from build123d import *

# Parameters (mm, degrees)
ESBO_O1_R                = 7.65
RESSALTO_EXTRUS_O1_DEPTH = 26
ESBO_O4_R                = 1.75
CORTE_EXTRUS_O1_DEPTH    = 20
ESBO_O5_W                = 3
ESBO_O5_H                = 5.6
CORTE_EXTRUS_O2_DEPTH    = 25
RESSALTO_EXTRUS_O2_DEPTH = 13
ESBO_O7_R                = 9
CORTE_EXTRUS_O3_DEPTH    = 10


with BuildPart() as part:
    # Esboço1 → Ressalto-extrusão1 (new body)
    with BuildSketch(Plane.XY):
        with BuildLine():
            Line((-7, 20.253205655), (-7, 18.253205655))
            Line((-7, 18.253205655), (-47, 18.253205655))
            Line((-47, 18.253205655), (-47, 8.253205655))
            Line((-47, 8.253205655), (-7, 8.253205655))
            Line((-7, 8.253205655), (-7, -20.253205655))
            ThreePointArc((-7, -20.253205655), (3.676851089, -41.422817781), (0, -18))
            Line((0, -18), (0, 18))
            ThreePointArc((0, 18), (3.676851089, 41.422817781), (-7, 20.253205655))
        make_face()
        with Locations(Location((0, 30, 0), (0, 0, 180))):
            Circle(ESBO_O1_R, mode=Mode.SUBTRACT)
        with Locations(Location((0, -30, 0), (0, 0, 180))):
            Circle(ESBO_O1_R, mode=Mode.SUBTRACT)
    extrude(amount=RESSALTO_EXTRUS_O1_DEPTH)

    # Esboço3 → Corte-Revolução1 (revolve, cut)
    with BuildSketch(Plane.ZY.offset(47)):
        Polygon((13, 18.253205655), (21, 18.253205655), (21, 15.753205655), (18.5, 15.753205655), (18.5, 10.753205655), (21, 10.753205655), (21, 8.253205655), (13, 8.253205655), align=None)
    revolve(axis=Axis((-47, 18.253205655, 13), (0, -1, 0)), mode=Mode.SUBTRACT)

    # Esboço4 → Corte-extrusão1 (cut)
    with BuildSketch(Plane.ZY.offset(47)):
        with Locations((5, 13.253205655)):
            Circle(ESBO_O4_R)
        with Locations(Location((21, 13.253205655, 0), (0, 0, 180))):
            Circle(ESBO_O4_R)
    extrude(amount=-CORTE_EXTRUS_O1_DEPTH, mode=Mode.SUBTRACT)

    # Esboço5 → Corte-extrusão2 (cut)
    with BuildSketch(Plane(origin=(0, 18.253205655, 0), x_dir=(1, 0, 0), z_dir=(0, 1, 0))):
        with Locations((-37, -5)):
            Rectangle(ESBO_O5_W, ESBO_O5_H)
        with Locations((-37, -21)):
            Rectangle(ESBO_O5_W, ESBO_O5_H)
    extrude(amount=-CORTE_EXTRUS_O2_DEPTH, mode=Mode.SUBTRACT)

    # Esboço6 → Ressalto-extrusão2 (add)
    with BuildSketch(Plane(origin=(0, 0, 0), x_dir=(0, 0, -1), z_dir=(1, 0, 0))):
        with BuildLine():
            Line((-17.5, -6), (-20.5, -6))
            ThreePointArc((-20.5, -6), (-23.5, -3), (-20.5, 0))
            Line((-20.5, 0), (-17.5, 0))
            ThreePointArc((-17.5, 0), (-14.5, -3), (-17.5, -6))
        make_face()
        with BuildLine():
            Line((-8.5, -6), (-5.5, -6))
            ThreePointArc((-5.5, -6), (-2.5, -3), (-5.5, 0))
            Line((-5.5, 0), (-8.5, 0))
            ThreePointArc((-8.5, 0), (-11.5, -3), (-8.5, -6))
        make_face()
    extrude(amount=RESSALTO_EXTRUS_O2_DEPTH)

    # Esboço7 → Corte-extrusão3 (cut)
    with BuildSketch(Plane(origin=(0, 18.253205655, 0), x_dir=(1, 0, 0), z_dir=(0, 1, 0))):
        with Locations(Location((-22, -13, 0), (0, 0, 180))):
            Circle(ESBO_O7_R)
    extrude(amount=-CORTE_EXTRUS_O3_DEPTH, mode=Mode.SUBTRACT)


solid = part.part
The model under review builds one solid part; all positions refer to its coordinate system, in mm. A direction names the side the tool comes from. Coordinates: 2 decimals unless noted, no trailing zeros. Loops run counter-clockwise (first coordinate to the right, second up) from the corner with the lowest first, then second, coordinate; pieces in that order, holes last.
(1) Consider section B-B, the plane x = -22. Give the boundary of the cut face in (y, z), plus the area to 3 significant figures.
Determined:
outline: (8.25, 0) - (18.25, 0) - (18.25, 4) - (8.25, 4) - close; (8.25, 22) - (18.25, 22) - (18.25, 26) - (8.25, 26) - close
area: 80.0 mm2
(2) Insertion check: P1, Ø13, axis at y = -2.5, z = 18.5, coming from the -X side; P2, Ø2.5, axis at x = 9.5, z = 7, coming from the -Y side; P3, Ø4, axis at x = -44, z = 16, coming from the +Y side; P4, Ø5, axis at x = -21, z = 19, coming from the +Y side. Each pin has a flat end and moves straight along its axis. Give the tip position at first contact, or say it passes through.
Determined:
P1: stops at x = -7
P2: stops at y = -38.71
P3: stops at y = 15.75
P4: passes through
(3) Draft analysis for pull direction Z (two halves, no side actions). For faces 1 (the flat face through (-27, 13, 5)), 2 (the cylindrical face through (0.996, -37.585, 12.818)), 3 (the flat face through (-6.7, 3.3, 0)), state which applies: +Z half, -Z half, draft (parallel to the pull), parting line (faces both ways), or undercut.
Determined:
face 1: undercut
face 2: draft
face 3: -Z half
(4) Consider section D-D, the plane y = -7. Give the boundary of the cut face in (x, z).
Determined:
outline: (-7, 0) - (0, 0) - (0, 26) - (-7, 26) - close
(5) Tool access review of faces 4 (the flat face through (-38.5, 13, 23)), 5 (the flat face through (-31.2, 18.253, 12.8)), 6 (the flat face through (6, -6, 19)), 7 (the cylindrical face through (-31.3, 14.3, 22.4)), 8 (the flat face through (-41, 10.753, 13)): name each direction out of +Z, -Z, +X, -X, +Y, -Y from which nothing blocks a thin tool from reaching the whole face with its end or side.
Determined:
face 4: +Y, -Y
face 5: +Z, -Z, -X
face 6: +Z, -Z, +X
face 7: -X
face 8: -X, -Y
(6) Consider section A-A, the plane z = 13. Give the boundary of the cut face in (x, y).
Determined:
outline: (-41.5, 10.75) - (-39, 10.75) - (-39, 8.25) - (-31, 8.25) - (-31, 18.25) - (-39, 18.25) - (-39, 15.75) - (-41.5, 15.75) - close; (-13, 8.25) - (-7, 8.25) - (-7, -20.25) arc R12 ccw (long way) to (0, -18) - (0, 18) arc R12 ccw (long way) to (-7, 20.25) - (-7, 18.25) - (-13, 18.25) - close; hole circle Ø15.3 at (0, -30); hole circle Ø15.3 at (0, 30)
(7) Consider section C-C, the plane y = -25. Give the boundary of the cut face in (x, z).
Determined:
outline: (-10.91, 0) - (-5.79, 0) - (-5.79, 26) - (-10.91, 26) - close; (5.79, 0) - (10.91, 0) - (10.91, 26) - (5.79, 26) - close
(8) Wall thickness on L1, parallel to Y at x = -32.5, z = 21; L2, parallel to Y at x = -11, z = 2.5; L3, parallel to Y at x = -4, z = 1.5: over which ranges is each line inside the solid? List them lowest first.
Determined:
L1: y = 8.25 to 11.5, 15 to 18.25
L2: y = -34.8 to -25.2, 8.25 to 18.25, 25.2 to 34.8
L3: y = -41.31 to -36.52, -23.48 to 23.48, 36.52 to 41.31
